from build123d import *

# Parameters (mm, degrees)
SKETCH_1_W            = 32.6
SKETCH_1_H            = 23.999999657
EXTRUDE_1_DEPTH       = 8.999999702
SKETCH_2_W            = 30.6
SKETCH_2_H            = 22
CUT_EXTRUDE_1_DEPTH   = 9.999999702
SKETCH_3_W            = 27.7
SKETCH_3_H            = 1.999999657
EXTRUDE_2_DEPTH       = 49.000000298
SKETCH_4_W            = 8.999999702
SKETCH_4_H            = 1.999999657
EXTRUDE_3_DEPTH       = 4.9
SKETCH_5_W            = 8.999999702
SKETCH_5_H            = 2
EXTRUDE_4_DEPTH       = 22
SKETCH_6_W            = 9
SKETCH_6_H            = 8
CUT_EXTRUDE_2_DEPTH   = 24.999999657
SKETCH_7_W            = 9
SKETCH_7_H            = 8
CUT_EXTRUDE_3_DEPTH   = 24.999999657
SKETCH_8_W            = 40
SKETCH_8_H            = 2
EXTRUDE_5_DEPTH       = 23.000000343
SKETCH_9_W            = 36.000000596
SKETCH_9_H            = 1.999999657
EXTRUDE_6_DEPTH       = 9
HOLE_WIZARD_4_0_4_1_D = 4
FILLET_1_R            = 2
SKETCH_12_R           = 1.897672249
SKETCH_12_R_2         = 2.0621459
CUT_EXTRUDE_4_DEPTH   = 2.999999657


with BuildPart() as part:
    # 草图1 → 凸台-拉伸1 (new body)
    with BuildSketch(Plane(origin=(29, 0, 0), x_dir=(0, 0, -1), z_dir=(1, 0, 0))):
        with Locations((-16.3, 13.000000171)):
            Rectangle(SKETCH_1_W, SKETCH_1_H)
    extrude(amount=-EXTRUDE_1_DEPTH)

    # 草图2 → 切除-拉伸1 (cut, through all)
    with BuildSketch(Plane.ZY.offset(-20.000000298)):
        with Locations((15.3, 12.000000343)):
            Rectangle(SKETCH_2_W, SKETCH_2_H)
    extrude(amount=-CUT_EXTRUDE_1_DEPTH, mode=Mode.SUBTRACT)

    # 草图3 → 凸台-拉伸2 (add)
    with BuildSketch(Plane.ZY.offset(-20.000000298)):
        with Locations((13.85, 24.000000171)):
            Rectangle(SKETCH_3_W, SKETCH_3_H)
    extrude(amount=EXTRUDE_2_DEPTH)

    # 草图4 → 凸台-拉伸3 (add)
    with BuildSketch(Plane.XY.offset(27.7)):
        with Locations((-24.500000149, 24.000000171)):
            Rectangle(SKETCH_4_W, SKETCH_4_H)
    extrude(amount=EXTRUDE_3_DEPTH)

    # 草图5 → 凸台-拉伸4 (add)
    with BuildSketch(Plane.XZ.offset(-23.000000343)):
        with Locations((-24.500000149, 31.6)):
            Rectangle(SKETCH_5_W, SKETCH_5_H)
    extrude(amount=EXTRUDE_4_DEPTH)

    # 草图6 → 切除-拉伸2 (cut, through all)
    with BuildSketch(Plane(origin=(0, 25, 0), x_dir=(-1, 0, 0), z_dir=(0, 1, 0))):
        with Locations((24.5, 4)):
            Rectangle(SKETCH_6_W, SKETCH_6_H)
    extrude(amount=-CUT_EXTRUDE_2_DEPTH, mode=Mode.SUBTRACT)

    # 草图7 → 切除-拉伸3 (cut, through all)
    with BuildSketch(Plane(origin=(0, 25, 0), x_dir=(-1, 0, 0), z_dir=(0, 1, 0))):
        with Locations((-24.5, 4)):
            Rectangle(SKETCH_7_W, SKETCH_7_H)
    extrude(amount=-CUT_EXTRUDE_3_DEPTH, mode=Mode.SUBTRACT)

    # 草图8 → 凸台-拉伸5 (add)
    with BuildSketch(Plane.XZ.offset(-23.000000343)):
        with Locations((0, 1)):
            Rectangle(SKETCH_8_W, SKETCH_8_H)
    extrude(amount=EXTRUDE_5_DEPTH)

    # 草图9 → 凸台-拉伸6 (add)
    with BuildSketch(Plane.XY.offset(27.7)):
        with Locations((0, 24.000000171)):
            Rectangle(SKETCH_9_W, SKETCH_9_H)
    extrude(amount=EXTRUDE_6_DEPTH)

    # Ø4.0 (4) 直径孔1 (through all)
    with Locations(Plane(origin=(0, 0, 30.6), x_dir=(-1, 0, 0), z_dir=(0, 0, -1))):
        with Locations((-24.75, 17.000000343), (-24.75, 7.000000343), (24.75, 17.000000343), (24.75, 7.000000343)):
            Hole(HOLE_WIZARD_4_0_4_1_D / 2)

    # 圆角1
    fillet_1_edges = [part.edges().sort_by_distance(p)[0] for p in [
        (-20, 0, 1),
        (20, 0, 1),
        (-18.000000298, 24.000000171, 36.7),
        (18.000000298, 24.000000171, 36.7),
        (-24.500000149, 25, 32.6),
        (-20.000000298, 1.000000343, 31.6),
        (-29, 1.000000343, 31.6),
        (29, 1.000000343, 31.6),
        (-29, 24.000000171, 8),
        (0, 25, 0),
        (24.500000149, 25, 32.6),
        (20.000000298, 1.000000343, 31.6),
        (29, 24.000000171, 8),
    ]]
    fillet(fillet_1_edges, radius=FILLET_1_R)

    # 草图12 → 切除-拉伸4 (cut, through all)
    with BuildSketch(Plane.XZ.offset(-23.000000343)):
        with Locations((-24.500000149, 24.8)):
            Circle(SKETCH_12_R)
        with Locations((-24.500000149, 14.8)):
            Circle(SKETCH_12_R_2)
        with Locations((24.500000149, 14.8)):
            Circle(SKETCH_12_R_2)
        with Locations((24.500000149, 24.8)):
            Circle(SKETCH_12_R)
    extrude(amount=-CUT_EXTRUDE_4_DEPTH, mode=Mode.SUBTRACT)


solid = part.part
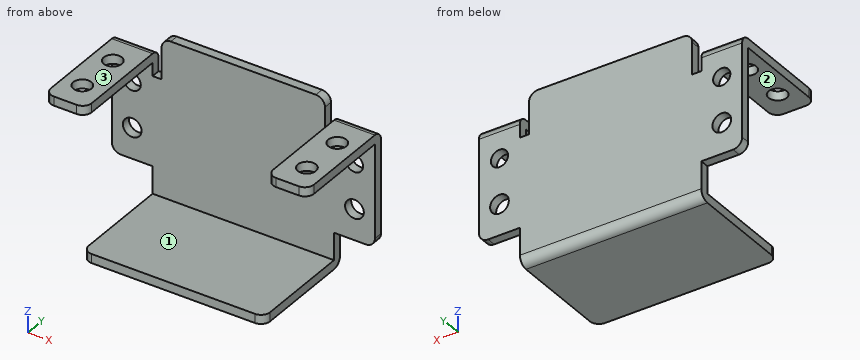
Design review of the part built by this model. Coordinates are the model's own, in mm. Face numbers are marked on the shaded views. A direction names the side the tool comes from. Round coordinates to 2 decimals unless told otherwise and drop trailing zeros. Loops run counter-clockwise (first coordinate to the right, second up) from the corner with the lowest first, then second, coordinate; pieces in that order, holes last. Notation, with made-up numbers: (24.5, -5) - (65.5, -5) arc R28 ccw to (65.5, 16) - close; hole circle Ø4 at (82, 33). An arc over 180 degrees is marked (long way). One line per item, written item: value. Start each with the question number.
1) Consider section C-C on y = 17. Give the boundary of the cut face in (x, z).
2) Consider section D-D on z = 32. Give the boundary of the cut face in (x, y).
3) To check wall thickness, follow L1, parallel to Y at x = 24, z = 31; L2, parallel to Z at x = -27, y = 4.75; L3, parallel to Z at x = 5, y = 16.25. State the ranges of each line that lie inside material, in increasing order. Write a range as from..to.
4) Consider section A-A on y = 11.5. Give the boundary of the cut face in (x, z), then the cut area to 3 significant figures.
5) Insertion check: pin 1 Ø2 at (x, y) = (24, 24.5) entering from -Z; pin 2 Ø12 at (x, y) = (8.5, 4) entering from +Z; pin 3 Ø6.5 at (x, z) = (-24.5, 14.8) entering from -Y. Each pin has a flat end and moves straight along its axis. Give the tip position at first contact, or say it passes through.
6) Consider section B-B on z = 14. Give the boundary of the cut face in (x, y), then the cut area to 3 significant figures.
7) For the marked faces 1, 2 and 3, list the 3-axis set-ups (+Z, -Z, +X, -X, +Y, -Y) from which the entire face can be reached by the end or side of a thin tool; tool diameter is ignored.
Reported:
1. outline: (-29, 30.6) - (-26.75, 30.6) - (-26.75, 32.6) - (-29, 32.6) - close; (-22.75, 30.6) - (-20, 30.6) - (-20, 32.6) - (-22.75, 32.6) - close; (-20, 0) - (20, 0) - (20, 2) - (-20, 2) - close; (20, 30.6) - (22.75, 30.6) - (22.75, 32.6) - (20, 32.6) - close; (26.75, 30.6) - (29, 30.6) - (29, 32.6) - (26.75, 32.6) - close
2. outline: (-29, 3) arc R2 ccw to (-27, 1) - (-22, 1) arc R2 ccw to (-20, 3) - (-20, 24.43) - (-29, 24.43) - close; (-18, 23) - (18, 23) - (18, 25) - (-18, 25) - close; (20, 3) arc R2 ccw to (22, 1) - (27, 1) arc R2 ccw to (29, 3) - (29, 24.43) - (20, 24.43) - close; hole circle Ø4 at (-24.75, 7); hole circle Ø4 at (-24.75, 17); hole circle Ø4 at (24.75, 7); hole circle Ø4 at (24.75, 17)
3. L1: y = 1..5.15, 8.85..15.15, 18.85..24.96
3. L2: z = 30.6..32.6
3. L3: z = 0..2
4. outline: (-29, 30.6) - (-20, 30.6) - (-20, 32.6) - (-29, 32.6) - close; (-20, 0) - (20, 0) - (20, 2) - (-20, 2) - close; (20, 30.6) - (29, 30.6) - (29, 32.6) - (20, 32.6) - close
4. area: 116 mm^2
5. pin 1: stops at z = 8
5. pin 2: stops at z = 2
5. pin 3: stops at y = 23
6. outline: (-29, 23) - (-26.4, 23) - (-26.4, 25) - (-29, 25) - close; (-22.6, 23) - (22.6, 23) - (22.6, 25) - (-22.6, 25) - close; (26.4, 23) - (29, 23) - (29, 25) - (26.4, 25) - close
6. area: 101 mm^2
7. face 1: +Z, +X, -X, -Y
7. face 2: -Z, +X, -X, -Y
7. face 3: +Z, +X, -X, +Y, -Y
